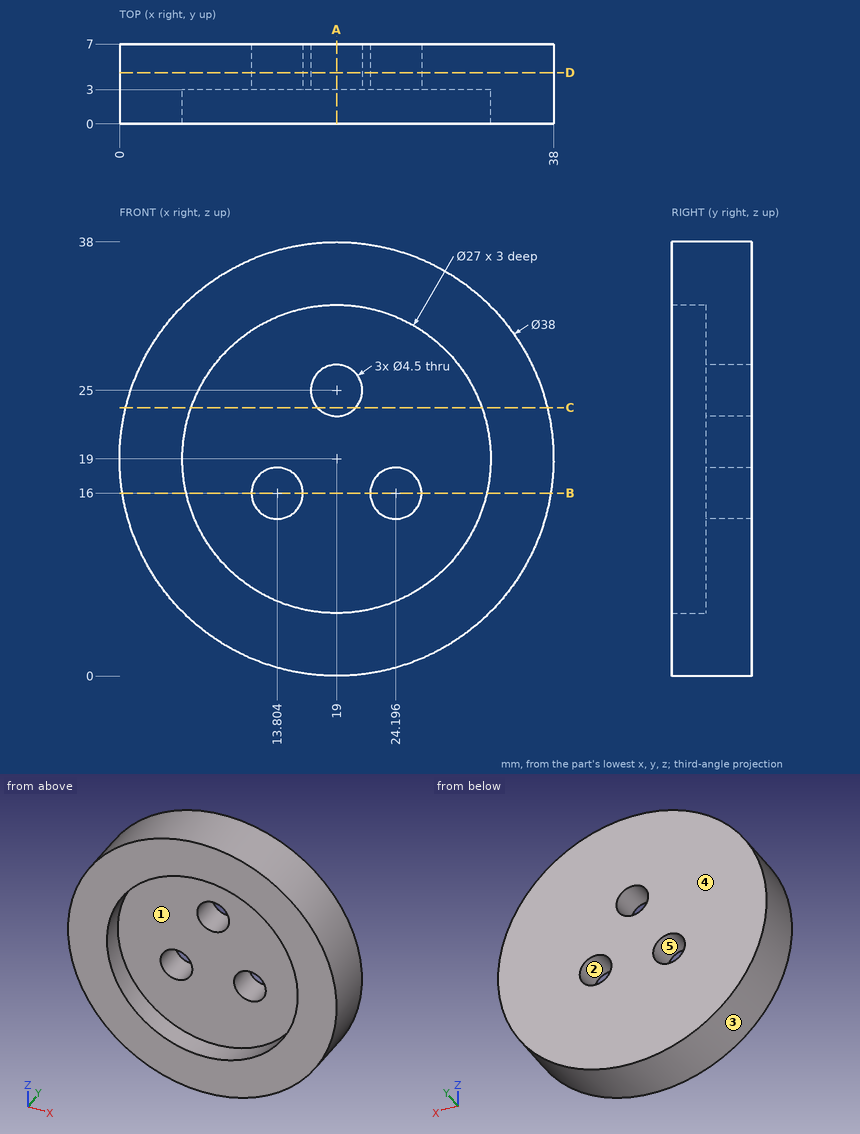
Can you work these out from the drawing? Everything is in mm from the part's minimum corner. A direction names the side the tool comes from. Coordinates: 2 decimals unless noted, no trailing zeros. Order: outer loops, then holes, each group sorted by start corner. A loop starts at its lowest first (then second) coordinate and runs counter-clockwise, first axis right, second up. Notation, with made-up numbers: M -11,40.25 L 17,40.25 A22 ccw 17,49.25 Z; hole C -4,78.5 d5. An arc over 180 degrees is marked long. Answer as CSV lines item,"result". Start each with the question number.
1. I want a section at C-C, the plane z = 23.5. Write out the boundary of the cut face in (x, y), and give its area (3 significant figures).
2. I need wall thicknesses on line 1 (X direction, y = 1.9, z = 19); line 2 (X direction, y = 1.75, z = 17); line 3 (Z direction, x = 23, y = 2.75). Which ranges of each line are inside material? Lowest first, please. Write a range as [from, to].
3. On a 3-axis mill with a long thin cutter (end or side, diameter ignored), from which of +Z, -Z, +X, -X, +Y, -Y can I reach the whole of each face in a straight line? I mean the marked faces 1 and 2. Say none if no direction works.
4. I want a section at D-D, the plane y = 4.5. Write out the boundary of the cut face in (x, z).
5. I want a section at A-A, the plane x = 19. Write out the boundary of the cut face in (y, z), and give its area (3 significant figures).
6. I want a section at B-B, the plane z = 16. Write out the boundary of the cut face in (x, y), and give its area (3 significant figures).
7. For pin 1 (2 mm diameter, centred on x = 15.5, z = 14, fed in from -Y); pin 2 (1 mm diameter, centred on x = 14, y = 3, fed in from +Z); pin 3 (2 mm diameter, centred on y = 3.5, z = 13, fed in from -X), each with a flat end and sliding along its axis, tell me the tip position at first contact or that it passes through.
8. We'd pull the mould along X, two halves only. Please class the marked faces 3, 4 and 5: released by +X, released by -X, zero draft, split by the parting line, or undercut.
Recorded:
1,outline,"M 0.54,0 L 6.27,0 L 6.27,3 L 17.32,3 L 17.32,7 L 0.54,7 Z; M 20.68,3 L 31.73,3 L 31.73,0 L 37.46,0 L 37.46,7 L 20.68,7 Z"
1,area,"169 mm2"
2,line 1,"x = [0, 5.5], [32.5, 38]"
2,line 2,"x = [0.11, 5.65], [32.35, 37.89]"
2,line 3,"z = [0.43, 6.11], [31.89, 37.57]"
3,face 1,"-Y"
3,face 2,"+Y, -Y"
4,outline,"C 19,19 d38; hole C 13.8,16 d4.5; hole C 19,25 d4.5; hole C 24.2,16 d4.5"
5,outline,"M 0,0 L 7,0 L 7,22.75 L 3,22.75 L 3,5.5 L 0,5.5 Z; M 0,32.5 L 3,32.5 L 3,27.25 L 7,27.25 L 7,38 L 0,38 Z"
5,area,"167 mm2"
6,outline,"M 0.24,0 L 5.84,0 L 5.84,3 L 11.55,3 L 11.55,7 L 0.24,7 Z; M 16.05,3 L 21.95,3 L 21.95,7 L 16.05,7 Z; M 26.45,3 L 32.16,3 L 32.16,0 L 37.76,0 L 37.76,7 L 26.45,7 Z"
6,area,"148 mm2"
7,pin 1,"stops at y = 3"
7,pin 2,"stops at z = 37.46"
7,pin 3,"stops at x = 0.67"
8,face 3,"split by the parting line"
8,face 4,"zero draft"
8,face 5,"undercut"
